Build history of the part. All positions in model axes, mm. Face numbers are marked on the shaded views. A direction names the side the tool comes from. Coordinates: 2 decimals unless noted, no trailing zeros. Order: outer loops, then holes, each group sorted by start corner. A loop starts at its lowest first (then second) coordinate and runs counter-clockwise, first axis right, second up. Notation, with made-up numbers: (48, 89) - (53, 89) arc R5 cw to (53, 95) - close; hole circle Ø4 at (3.25, 50.5). An arc over 180 degrees is marked (long way). Answer as CSV lines item,"result". Start each with the question number.
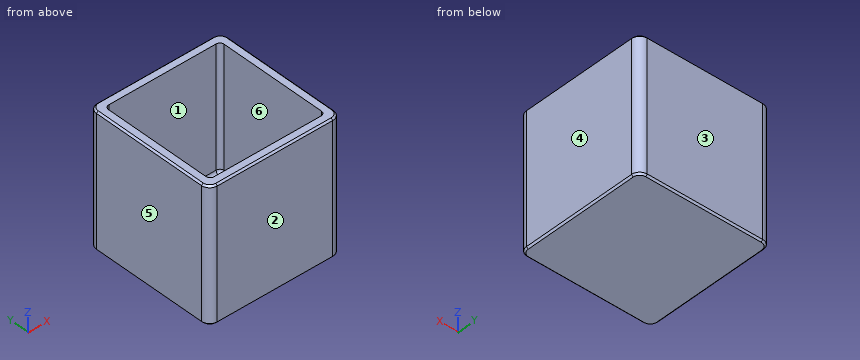
from build123d import *

# Parameters (mm, degrees)
F1_DEPTH = 80
F2_T     = 5
F3_R     = 2.5
F4_SIZE  = 1


# Not quite as in the source:
# - a shell that OpenCascade refuses in one call is made with other operations: the cavity is built on its own and cut out


with BuildPart() as f1:
    # F0 (on Top) → F1 (new body)
    with BuildSketch(Plane.XY):
        with BuildLine():
            Line((35, 40), (-35, 40))
            ThreePointArc((-35, 40), (-38.5355339059, 38.5355339059), (-40, 35))
            Line((-40, 35), (-40, -35))
            ThreePointArc((-40, -35), (-38.5355339059, -38.5355339059), (-35, -40))
            Line((-35, -40), (35, -40))
            ThreePointArc((35, -40), (38.5355339059, -38.5355339059), (40, -35))
            Line((40, -35), (40, 35))
            ThreePointArc((40, 35), (38.5355339059, 38.5355339059), (35, 40))
        make_face()
    extrude(amount=F1_DEPTH)

    # F2: shell of thickness 5, made by hand


with BuildPart() as f2_core1:
    # F2_t2: copy of F1
    add(f1.part)

    # the walls: a layer under each face that stays
    f2_faces = [f2_core1.faces().sort_by_distance(p)[0] for p in [
        (0, 40, 40),
        (-40, 0, 40),
        (0, -40, 40),
        (40, 0, 40),
        (0, 0, 0),
    ]]
    thicken(f2_faces, amount=-F2_T, mode=Mode.SUBTRACT)


with BuildPart() as f1_1:
    add(f1.part)

    # what is left inside the walls is the cavity
    f2_cavity = [f2_core1.part.solids().sort_by_distance(p)[0] for p in [
        (0, 34.95, 55),
    ]]
    add(f2_cavity, mode=Mode.SUBTRACT)

    # F3
    f3_edges = [f1_1.edges().sort_by_distance(p)[0] for p in [
        (35, 35, 42.5),
        (-35, 35, 42.5),
        (-35, -35, 42.5),
        (35, -35, 42.5),
        (35, 0, 5),
        (0, -35, 5),
        (-35, 0, 5),
        (0, 35, 5),
    ]]
    fillet(f3_edges, radius=F3_R)

    # F4
    f4_edges = [f1_1.edges().sort_by_distance(p)[0] for p in [
        (0, 40, 0),
        (-38.535534, 38.535534, 0),
        (-40, 0, 0),
        (-38.535534, -38.535534, 0),
        (0, -40, 0),
        (38.535534, -38.535534, 0),
        (40, 0, 0),
        (38.535534, 38.535534, 0),
        (0, 40, 80),
        (-38.535534, 38.535534, 80),
    ]]
    chamfer(f4_edges, length=F4_SIZE)


solid = f1_1.part
(1) Pull direction X, two halves, no side cores. Call the marked faces 3, 4, 5 and 6: +X half, -X half, draft (parallel to the pull), parting line (faces both ways), or undercut.
(2) Which spindle directions (+Z, -Z, +X, -X, +Y, -Y) get a long thin tool onto all of the face, cutting with end or side? Do the marked faces 1 and 2. Say none if no direction does.
(3) Probe L1, parallel to X at y = 8.5, z = 18; L2, parallel to Z at x = 27.5, y = -8.5. List the from-to ranges inside material, lowest first. Write a range as [from, to].
(4) Drop a flat-ended pin along its axis: pin 1 Ø5 at (x, y) = (-28, -6.5) entering from +Z. Give the stop position or say it passes through.
(5) Band-saw the part on A-A on z = 45.5. List the corners of the cut face in (x, y).
(6) Band-saw the part on B-B on x = 14. List the corners of the cut face in (y, z), plus the area to 3 significant figures.
Filled in:
1,face 3,"draft"
1,face 4,"+X half"
1,face 5,"-X half"
1,face 6,"undercut"
2,face 1,"+Z"
2,face 2,"+Z, -Z, +X, -X, -Y"
3,L1,"x = [-40, -35], [35, 40]"
3,L2,"z = [0, 5]"
4,pin 1,"stops at z = 5"
5,outline,"(-40, -35) arc R5 ccw to (-35, -40) - (35, -40) arc R5 ccw to (40, -35) - (40, 35) arc R5 ccw to (35, 40) - (-35, 40) arc R5 ccw to (-40, 35) - close; hole (-35, -32.5) arc R2.5 ccw to (-32.5, -35) - (32.5, -35) arc R2.5 ccw to (35, -32.5) - (35, 32.5) arc R2.5 ccw to (32.5, 35) - (-32.5, 35) arc R2.5 ccw to (-35, 32.5) - close"
6,outline,"(-40, 1) - (-39, 0) - (39, 0) - (40, 1) - (40, 79) - (39, 80) - (35, 80) - (35, 7.5) arc R2.5 cw to (32.5, 5) - (-32.5, 5) arc R2.5 cw to (-35, 7.5) - (-35, 80) - (-39, 80) - (-40, 79) - close"
6,area,"1,150 mm^2"
